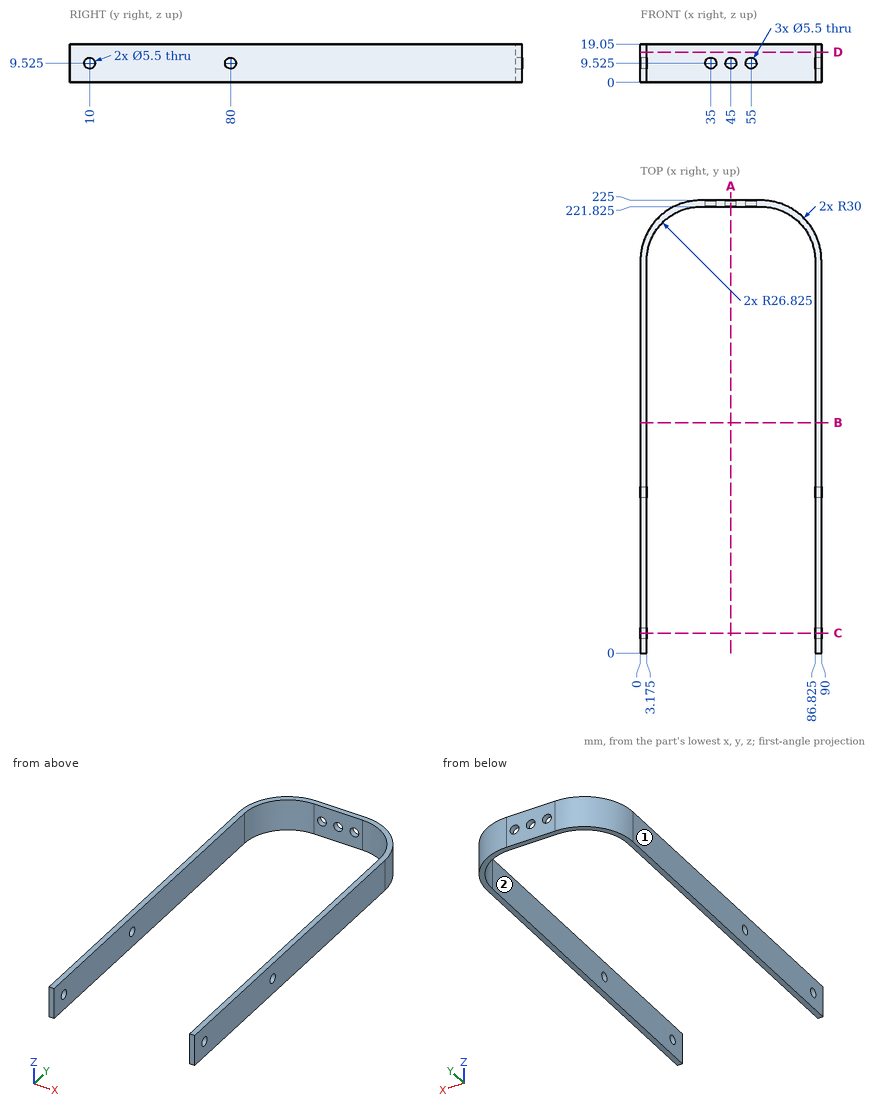
Geometry check sheet. Reference: drawing and pictorial views, mm from the part's lowest x, y, z. A direction names the side the tool comes from. Give positions to 0.01 mm unless a question says otherwise; leave off trailing zeros. Order: outer loops, then holes, each group sorted by start corner. A loop starts at its lowest first (then second) coordinate and runs counter-clockwise, first axis right, second up. Notation, with made-up numbers: M 34.5,-40 L 83.5,-40 A12 ccw 83.5,-28 Z; hole C -33.75,-10 d6. An arc over 180 degrees is marked long. Return JSON: item names as keys, results as strings. Group by question number.
1) Section check D-D on z = 15. Record the cut outline in (x, y) (3 decimals).
2) Section check B-B on y = 114.5. Record the cut outline in (x, z) (3 decimals).
3) Section check A-A on x = 45. Record the cut outline in (y, z) (3 decimals), and give its area (3 significant figures).
4) Access from +Z, -Z, +X, -X, +Y, -Y to the whole of each face (thin tool, end or side, straight path). Record for the marked faces 1 and 2.
5) Section check C-C on y = 10. Record the cut outline in (x, z) (3 decimals), and give its area (3 significant figures).
6) Scan lines: line 1 (X direction, y = 135, z = 6.5) (3 decimals); line 2 (Z direction, x = 2, y = 80) (3 decimals); line 3 (X direction, y = 202, z = 2.75). Record each from-to range of solid material in increasing order.
7) Go/stop test with flat-tipped pins: pin 1 Ø7 at (y, z) = (80, 9.525) entering from +X; pin 2 Ø5.5 at (x, z) = (46.5, 13.5) entering from -Y (3 decimals); pin 3 Ø6 at (x, z) = (25.5, 7.5) entering from +Y. Record where each tip stops, or that it passes through.
Answer block:
{
 "1": {"outline": "M 0,0 L 3.175,0 L 3.175,195 A26.825 cw 30,221.825 L 60,221.825 A26.825 cw 86.825,195 L 86.825,0 L 90,0 L 90,195 A30 ccw 60,225 L 30,225 A30 ccw 0,195 Z"},
 "2": {"outline": "M 0,0 L 3.175,0 L 3.175,19.05 L 0,19.05 Z; M 86.825,0 L 90,0 L 90,19.05 L 86.825,19.05 Z"},
 "3": {"outline": "M 221.825,0 L 225,0 L 225,6.775 L 221.825,6.775 Z; M 221.825,12.275 L 225,12.275 L 225,19.05 L 221.825,19.05 Z", "area": "43.0 mm^2"},
 "4": {"face 1": "+Z, -Z, -X, +Y, -Y", "face 2": "+Z, -Z, -Y"},
 "5": {"outline": "M 0,0 L 3.175,0 L 3.175,6.775 L 0,6.775 Z; M 0,12.275 L 3.175,12.275 L 3.175,19.05 L 0,19.05 Z; M 86.825,0 L 90,0 L 90,6.775 L 86.825,6.775 Z; M 86.825,12.275 L 90,12.275 L 90,19.05 L 86.825,19.05 Z", "area": "86.0 mm^2"},
 "6": {"line 1": "x = 0 to 3.175, 86.825 to 90", "line 2": "z = 0 to 6.775, 12.275 to 19.05", "line 3": "x = 0.83 to 4.1, 85.9 to 89.17"},
 "7": {"pin 1": "stops at x = 90", "pin 2": "stops at y = 221.825", "pin 3": "stops at y = 224.96"}
}
